Geometry check sheet. Reference: the model listing, model coordinates, mm. A direction names the side the tool comes from. Coordinates: 2 decimals unless noted, no trailing zeros. Order: outer loops, then holes, each group sorted by start corner. A loop starts at its lowest first (then second) coordinate and runs counter-clockwise, first axis right, second up. Notation, with made-up numbers: (-13.75, -26) - (21.25, -26) arc R23 ccw to (21.25, 1) - close; hole circle Ø6 at (3.5, -1). An arc over 180 degrees is marked (long way). Use CSV: the item, a comma, the result in double quotes. Start each with the question number.
1) Sectioned sample at B-B, the plane z = 4. Count the separate pieces of the cut face and the enclosed holes in it, and give its area (3 significant figures).
2) Tool access check on faces 1 (the cylindrical face through (-26.75, -103.21, 4.93)), 2 (the flat face through (-85, -2, 5)). Record the directions out of +Z, -Z, +X, -X, +Y, -Y that give a thin tool (end or side, any length) a straight path to the whole face; none if there is none.
3) Thickness scan on probe 1 along Y at (x, z) = (50, 2.75); probe 2 along X at (y, z) = (-63.5, 2.75); probe 3 along Y at (x, z) = (63.5, 0.5). Record the ranges inside material, lowest first. Write a range as [from, to].
4) Draft check along Y on faces 3 (the flat face through (-46, 99.563, 5)), 4 (the flat face through (-1, -115, 5)), 5 (the flat face through (85, -2, 5)). Enter one of: released by +Y, released by -Y, zero draft, split by the parting line, or undercut.
5) Sectioned sample at A-A, the plane x = -40.5. Record the cut outline in (y, z), and give its area (3 significant figures).
6) Depth check by flat-ended pin: P1, Ø12, axis at x = -56.5, y = -85, coming from the -Z side. Enter the tip coordinate at first touch or a pass-through.
from build123d import *

# Parameters (mm, degrees)
SKETCH1_W           = 170
SKETCH1_H           = 230
BOSS_EXTRUDE1_DEPTH = 10


with BuildPart() as part:
    # Sketch1 → Boss-Extrude1 (new body)
    with BuildSketch(Plane.XY):
        Rectangle(SKETCH1_W, SKETCH1_H)
        with BuildLine():
            Line((30.314685315, 106.695804196), (60.314685315, 106.695804196))
            ThreePointArc((60.314685315, 106.695804196), (63.881118881, 103.129370629), (60.314685315, 99.562937063))
            Line((60.314685315, 99.562937063), (30.314685315, 99.562937063))
            ThreePointArc((30.314685315, 99.562937063), (26.748251748, 103.129370629), (30.314685315, 106.695804196))
        make_face(mode=Mode.SUBTRACT)
        with BuildLine():
            Line((35, -75), (35, -65))
            ThreePointArc((35, -65), (32.5, -62.5), (30, -65))
            Line((30, -65), (30, -75))
            ThreePointArc((30, -75), (32.5, -77.5), (35, -75))
        make_face(mode=Mode.SUBTRACT)
        with BuildLine():
            Line((-30.314685315, 106.695804196), (-60.314685315, 106.695804196))
            ThreePointArc((-60.314685315, 106.695804196), (-63.881118881, 103.129370629), (-60.314685315, 99.562937063))
            Line((-60.314685315, 99.562937063), (-30.314685315, 99.562937063))
            ThreePointArc((-30.314685315, 99.562937063), (-26.748251748, 103.129370629), (-30.314685315, 106.695804196))
        make_face(mode=Mode.SUBTRACT)
        with BuildLine():
            Line((30, 21), (30, 11))
            ThreePointArc((30, 11), (32.5, 8.5), (35, 11))
            Line((35, 11), (35, 21))
            ThreePointArc((35, 21), (32.5, 23.5), (30, 21))
        make_face(mode=Mode.SUBTRACT)
        with BuildLine():
            Line((-30, 21), (-30, 11))
            ThreePointArc((-30, 11), (-32.5, 8.5), (-35, 11))
            Line((-35, 11), (-35, 21))
            ThreePointArc((-35, 21), (-32.5, 23.5), (-30, 21))
        make_face(mode=Mode.SUBTRACT)
        with BuildLine():
            Line((-30, -75), (-30, -65))
            ThreePointArc((-30, -65), (-32.5, -62.5), (-35, -65))
            Line((-35, -65), (-35, -75))
            ThreePointArc((-35, -75), (-32.5, -77.5), (-30, -75))
        make_face(mode=Mode.SUBTRACT)
        with BuildLine():
            Line((-30.314685315, -99.562937063), (-60.314685315, -99.562937063))
            ThreePointArc((-60.314685315, -99.562937063), (-63.881118881, -103.129370629), (-60.314685315, -106.695804196))
            Line((-60.314685315, -106.695804196), (-30.314685315, -106.695804196))
            ThreePointArc((-30.314685315, -106.695804196), (-26.748251748, -103.129370629), (-30.314685315, -99.562937063))
        make_face(mode=Mode.SUBTRACT)
        with BuildLine():
            Line((30.314685315, -99.562937063), (60.314685315, -99.562937063))
            ThreePointArc((60.314685315, -99.562937063), (63.881118881, -103.129370629), (60.314685315, -106.695804196))
            Line((60.314685315, -106.695804196), (30.314685315, -106.695804196))
            ThreePointArc((30.314685315, -106.695804196), (26.748251748, -103.129370629), (30.314685315, -99.562937063))
        make_face(mode=Mode.SUBTRACT)
    extrude(amount=BOSS_EXTRUDE1_DEPTH)


solid = part.part
Evaluation:
1,separate pieces,"1"
1,enclosed holes,"8"
1,area,"37,800 mm²"
2,face 1,"+Z, -Z"
2,face 2,"+Z, -Z, -X, +Y, -Y"
3,probe 1,"[-115, -106.7], [-99.56, 99.56], [106.7, 115]"
3,probe 2,"[-85, -34.5], [-30.5, 30.5], [34.5, 85]"
3,probe 3,"[-115, -104.73], [-101.53, 101.53], [104.73, 115]"
4,face 3,"undercut"
4,face 4,"released by -Y"
4,face 5,"zero draft"
5,outline,"(-115, 0) - (-106.7, 0) - (-106.7, 10) - (-115, 10) - close; (-99.56, 0) - (99.56, 0) - (99.56, 10) - (-99.56, 10) - close; (106.7, 0) - (115, 0) - (115, 10) - (106.7, 10) - close"
5,area,"2,160 mm²"
6,P1,"z = 0"
